Model file for the job. Use its own axes, mm. Coordinates: 2 decimals unless noted, no trailing zeros. Order: outer loops, then holes, each group sorted by start corner. A loop starts at its lowest first (then second) coordinate and runs counter-clockwise, first axis right, second up. Notation, with made-up numbers: (-9.5, 38.25) -> (5.5, 38.25) arc R22 cw to (5.5, 45.25) -> close; hole circle Ø7 at (66, 71.25). An arc over 180 degrees is marked (long way). Use CSV: the item, a comma, the result in double quotes. Start each with the question number.
(1) Cut at A-A on z = 1. Write the cut outline in (x, y).
(2) Cut at B-B on z = 3.75. Write the cut outline in (x, y).
(3) Probe L1, parallel to X at y = 0, z = 4.1; L2, parallel to Y at x = 0, z = 4.15; L3, parallel to Y at x = 0, z = 2.8. List the from-to ranges inside material, lowest first.
(4) Pin check, flat tips, straight feed: pin 1 Ø3 at (x, y) = (4.5, 6) entering from +Z; pin 2 Ø1.5 at (x, z) = (0.5, 3) entering from -Y; pin 3 Ø6 at (x, y) = (3.5, -7.5) entering from +Z. Stop position of each tip, or through.
(5) Pull direction X, two halves, no side cores. Call faces 1 (the flat face through (3, 2, 0)), 2 (the cylindrical face through (2.539, 1.947, 2.712)), 3 (the conical face through (-2.957, -4.638, 5.675)): pulls with the +X half, pulls with the -X half, needs draft (parallel to the pull), parting line crosses it, or undercut.
```python
from build123d import *

# Parameters (mm, degrees)
F2_R    = 2
F3_SIZE = 0.5


with BuildPart() as f1:
    # F0 (on Front) → F1 (revolve)
    with BuildSketch(Plane.XZ):
        Polygon((-11, 0), (-3.2, 0), (-3.2, 5.848632), (-5.2, 5.848632), (-11, 2.5), align=None)
    revolve(axis=Axis((0, 0, 13.586091), (0, 0, 1)))

    # F2
    f2_edges = [f1.edges().sort_by_distance(p)[0] for p in [
        (11, 0, 2.5),
    ]]
    fillet(f2_edges, radius=F2_R)

    # F3
    f3_edges = [f1.edges().sort_by_distance(p)[0] for p in [
        (3.2, 0, 5.848632),
    ]]
    chamfer(f3_edges, length=F3_SIZE)


solid = f1.part
```
Outcome:
1,outline,"circle Ø22 at (0, 0); hole circle Ø6.4 at (0, 0)"
2,outline,"circle Ø17.67 at (0, 0); hole circle Ø6.4 at (0, 0)"
3,L1,"-8.23 to -3.2, 3.2 to 8.23"
3,L2,"-8.14 to -3.2, 3.2 to 8.14"
3,L3,"-10.37 to -3.2, 3.2 to 10.37"
4,pin 1,"z = 5.39"
4,pin 2,"y = -10.77"
4,pin 3,"z = 5.8"
5,face 1,"needs draft"
5,face 2,"undercut"
5,face 3,"parting line crosses it"
